The listing builds one solid part. Answer for the finished solid, in the listing's coordinates (mm). A direction names the side the tool comes from. Give positions to 0.01 mm unless a question says otherwise; leave off trailing zeros. Loops run counter-clockwise (first coordinate to the right, second up) from the corner with the lowest first, then second, coordinate; pieces in that order, holes last. Notation, with made-up numbers: M 50,85.25 L 100,85.25 A22 cw 100,107.25 Z; hole C 50,-28 d6. An arc over 180 degrees is marked long. Use one line per item in the form item = value. Start each with the question number.
1. Straight lines are drawn through the part: line 1 (Y direction, x = 0, z = -0.5); line 2 (Z direction, x = 20, y = 4.75); line 3 (Y direction, x = -2.5, z = 3). For each, find the intervals that lie inside material, in ascending order. Write a range as from..to.
2. Each of these flat-tipped pins is pushed along its axis until it touches: pin 1 Ø4 at (x, z) = (-20, 0) entering from +Y; pin 2 Ø9 at (x, y) = (0, 0) entering from -Z. Where does it stop, or does it pass through?
3. The part is cut by section B-B (x = 0). Write down the section's boundary in (y, z).
4. The part is cut by section D-D (y = 11). Write down the section's boundary in (x, z), and give its area (3 significant figures).
5. For faces 5 (the face through (-22.003, 4.86, -0.631)), 6 (the face through (-27.5, 0, 0)), determine the directions among +Z, -Z, +X, -X, +Y, -Y from which every point of the face is accessible in a straight line to the end or side of a thin tool.
6. The part is cut by section C-C (z = 5.5). Write down the section's boundary in (x, y).
7. The mould has two halves that part along Z. Classify faces 1 (the face through (17.997, 4.86, -0.631)), 2 (the face through (0, -15, 0)), 3 (the face through (-6, 0, -7.5)), 4 (the face through (-20.364, -6.043, -0.016)): released by +Z, released by -Z, zero draft, split by the parting line, or undercut.
8. The part is cut by section A-A (y = 0). Write down the section's boundary in (x, z).
from build123d import *

# Parameters (mm, degrees)
SKETCH1_W             = 55
SKETCH1_H             = 15
BOSS_EXTRUDE1_DEPTH   = 15
SKETCH3_R             = 5
CUT_EXTRUDE1_DEPTH    = 35.731109974
M5_TAPPED_HOLE1_D     = 4.2
M5_TAPPED_HOLE1_DEPTH = 20
M5_TAPPED_HOLE1_TIP   = 1.2618073


with BuildPart() as part:
    # Sketch1 → Boss-Extrude1 (new, symmetric)
    with BuildSketch(Plane(origin=(0, 0, 0), x_dir=(1, 0, 0), z_dir=(0, 1, 0))):
        Rectangle(SKETCH1_W, SKETCH1_H)
    extrude(amount=BOSS_EXTRUDE1_DEPTH, both=True)

    # Sketch3 → Cut-Extrude1 (cut, through all)
    with BuildSketch(Plane.XY.offset(7.5)):
        Circle(SKETCH3_R)
    extrude(amount=-CUT_EXTRUDE1_DEPTH, mode=Mode.SUBTRACT)

    # M5 Tapped Hole1
    with Locations(Plane(origin=(0, 15, 0), x_dir=(1, 0, 0), z_dir=(0, 1, 0))):
        with Locations((-20, 0), (20, 0)):
            Hole(M5_TAPPED_HOLE1_D / 2, depth=M5_TAPPED_HOLE1_DEPTH)
            with Locations((0, 0, -(M5_TAPPED_HOLE1_DEPTH + M5_TAPPED_HOLE1_TIP / 2))):  # 118° drill point
                Cone(0, M5_TAPPED_HOLE1_D / 2, M5_TAPPED_HOLE1_TIP, mode=Mode.SUBTRACT)


solid = part.part
Derived:
q1.line_1 = -15..-5, 5..15
q1.line_2 = -7.5..-2.1, 2.1..7.5
q1.line_3 = -15..-4.33, 4.33..15
q2.pin_1 = -5.06
q2.pin_2 = through
q3.outline = M -15,-7.5 L -5,-7.5 L -5,7.5 L -15,7.5 Z; M 5,-7.5 L 15,-7.5 L 15,7.5 L 5,7.5 Z
q4.outline = M -27.5,-7.5 L 27.5,-7.5 L 27.5,7.5 L -27.5,7.5 Z; hole C -20,0 d4.2; hole C 20,0 d4.2
q4.area = 797 mm2
q5.face_5 = +Y
q5.face_6 = +Z, -Z, -X, +Y, -Y
q6.outline = M -27.5,-15 L 27.5,-15 L 27.5,15 L -27.5,15 Z; hole C 0,0 d10
q7.face_1 = undercut
q7.face_2 = zero draft
q7.face_3 = released by -Z
q7.face_4 = undercut
q8.outline = M -27.5,-7.5 L -5,-7.5 L -5,7.5 L -27.5,7.5 Z; M 5,-7.5 L 27.5,-7.5 L 27.5,7.5 L 5,7.5 Z; hole C -20,0 d4.2; hole C 20,0 d4.2
